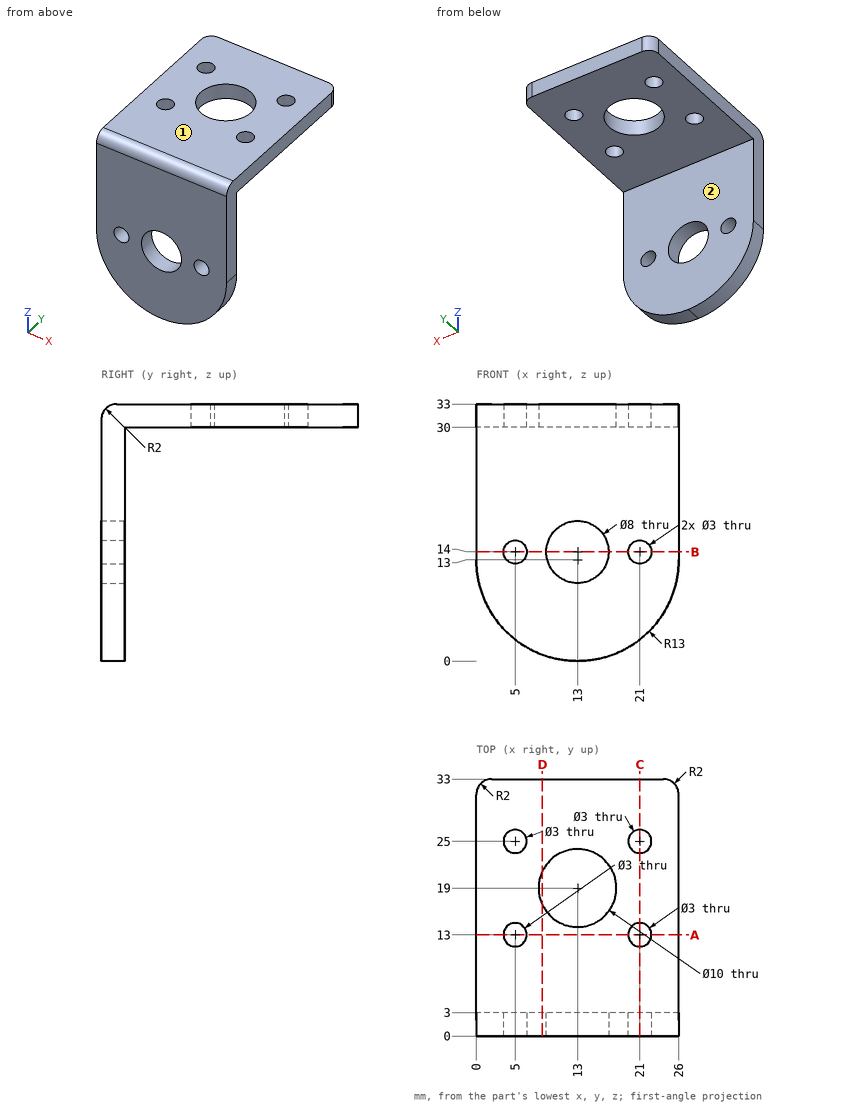
Design review of the part shown in the three views and the two pictorial views. Dimensions are in mm from the part's minimum x, y and z. A direction names the side the tool comes from. Give positions to 0.01 mm unless a question says otherwise; leave off trailing zeros. Loops run counter-clockwise (first coordinate to the right, second up) from the corner with the lowest first, then second, coordinate; pieces in that order, holes last. Notation, with made-up numbers: M 16,49 L 54,49 A12 cw 54,63 Z; hole C -31,17.25 d4. An arc over 180 degrees is marked long. Write item = value, one per line.
Q1. Insertion check: pin 1 (2.5 mm diameter, centred on x = 5, y = 13, fed in from +Z); pin 2 (6 mm diameter, centred on x = 16.5, z = 6, fed in from -Y); pin 3 (1.5 mm diameter, centred on x = 18, y = 15, fed in from -Z); pin 4 (3 mm diameter, centred on x = 12.5, z = 4.5, fed in from +Y). Each pin has a flat end and moves straight along its axis. Give the tip position at first contact, or say it passes through.
Output values:
pin_1 = through
pin_2 = 0
pin_3 = 30
pin_4 = 3
Q2. For the marked faces 1 and 2, list the 3-axis set-ups (+Z, -Z, +X, -X, +Y, -Y) from which the entire face can be reached by the end or side of a thin tool; tool diameter is ignored.
Output values:
face_1 = +Z, +X, -X, +Y, -Y
face_2 = -Z, +X, -X, +Y
Q3. We need section B-B (z = 14). Give the boundary of the cut face in (x, y), plus the area to 3 significant figures.
Output values:
outline = M 0,0 L 3.5,0 L 3.5,3 L 0,3 Z; M 6.5,0 L 9,0 L 9,3 L 6.5,3 Z; M 17,0 L 19.5,0 L 19.5,3 L 17,3 Z; M 22.5,0 L 26,0 L 26,3 L 22.5,3 Z
area = 36.0 mm^2
Q4. To check wall thickness, follow line 1 (X direction, y = 1, z = 14); line 2 (Y direction, x = 21, z = 31); line 3 (Y direction, x = 21, z = 31.45). State the ranges of each line that lie inside material, in increasing order. Write a range as [from, to].
Output values:
line_1 = [0, 3.5], [6.5, 9], [17, 19.5], [22.5, 26]
line_2 = [0, 11.5], [14.5, 23.5], [26.5, 33]
line_3 = [0.05, 11.5], [14.5, 23.5], [26.5, 33]
Q5. We need section A-A (y = 13). Give the boundary of the cut face in (x, z), plus the area to 3 significant figures.
Output values:
outline = M 0,30 L 3.5,30 L 3.5,33 L 0,33 Z; M 6.5,30 L 19.5,30 L 19.5,33 L 6.5,33 Z; M 22.5,30 L 26,30 L 26,33 L 22.5,33 Z
area = 60.0 mm^2
Q6. We need section D-D (x = 8.5). Give the boundary of the cut face in (y, z).
Output values:
outline = M 0,0.8 L 3,0.8 L 3,30 L 16.82,30 L 16.82,33 L 2,33 A2 ccw 0,31 Z; M 21.18,30 L 33,30 L 33,33 L 21.18,33 Z
Q7. We need section C-C (x = 21). Give the boundary of the cut face in (y, z).
Output values:
outline = M 0,2.75 L 3,2.75 L 3,12.5 L 0,12.5 Z; M 0,15.5 L 3,15.5 L 3,30 L 11.5,30 L 11.5,33 L 2,33 A2 ccw 0,31 Z; M 14.5,30 L 23.5,30 L 23.5,33 L 14.5,33 Z; M 26.5,30 L 33,30 L 33,33 L 26.5,33 Z
